Geometry: final body of the model. Coordinates: model frame, mm. A direction names the side the tool comes from. Coordinates: 2 decimals unless noted, no trailing zeros. Write each loop counter-clockwise with the first axis right and the second up, starting at its lowest first coordinate (ties: lowest second). Pieces come first, ordered by that corner, then holes. Notation, with made-up numbers: M 15,6 L 38,6 A28 cw 38,26 Z; hole C 85.25,-36 d2. An arc over 180 degrees is marked long. Write item = value, one per line. Start each with the question number.
Item 1: Pull-direction query (Z, two-part tool) for faces 6 (the flat face through (-119, 24, -155.575)), 7 (the flat face through (0, 19, 5)), 8 (the flat face through (-241.3, 5, -163)), 9 (the flat face through (-119, 22, -152.4)); classes: +Z half, -Z half, draft (parallel to the pull), parting line (faces both ways), or undercut.
Item 2: First-contact query: pin 1 Ø17.5 at (x, y) = (-103.5, 19) entering from -Z (3 decimals); pin 2 Ø3.5 at (y, z) = (39, -153.5) entering from +X (3 decimals); pin 3 Ø8.5 at (x, y) = (-228.6, 28.575) entering from +Z; pin 4 Ø1.5 at (x, y) = (-41, 23) entering from +Z (3 decimals). Flat tips, straight axial feed; report the tip coordinate or a pass-through.
Item 3: Reachability of faces 1 (the flat face through (-119, 3.175, -172)), 2 (the flat face through (-119, 24, 155.575)), 3 (the flat face through (20, 3.175, 5)), 4 (the flat face through (-119, 6.35, -173)), 5 (the flat face through (-119, 22, 152.4)) from +Z, -Z, +X, -X, +Y, -Y: full face, straight path, thin tool, end or side. Return the list, or none.
Item 4: Section B-B on z = 2.5. Output: boundary loops of the cut face in (x, y) (3 decimals), plus the area to 3 significant figures.
Item 5: Section A-A on x = -106.5. Output: boundary loops of the cut face in (y, z) (3 decimals).
Item 6: Ray query, L1, parallel to Z at x = -228.6, y = 4.1 (3 decimals); L2, parallel to Z at x = 25, y = 1; L3, parallel to Z at x = -209.5, y = 22 (3 decimals). Return the intervals inside material, ascending. Write a range as [from, to].
from build123d import *

# Parameters (mm, degrees)
EXTRUDE_THIN1_DEPTH     = 342.9
EXTRUDE_THIN2_DEPTH     = 241.3
CUT_EXTRUDE1_REACH      = 423.02
SKETCH3_R               = 3.175
CUT_EXTRUDE2_REACH      = 423.319
SKETCH4_R               = 3.175
CUT_EXTRUDE3_DEPTH      = 422.319030694
CUT_EXTRUDE3_DEPTH_BACK = 422.319030694
SKETCH5_R               = 4.7625


# Read off the part's stored shape, not the designer's step: Extrude-Thin2
with BuildPart() as part:
    # Sketch1 → Extrude-Thin1 (new, symmetric)
    with BuildSketch(Plane.XY):
        Polygon((38.1, 0), (0, 0), (0, 38.1), (3.175, 38.1), (3.175, 3.175), (38.1, 3.175), align=None)
    extrude(amount=EXTRUDE_THIN1_DEPTH, both=True)

    # Extrude-Thin2 outline → Extrude-Thin2 (add)
    with BuildSketch(Plane.ZY):
        Polygon((-152.4, 3.175), (-152.4, 41.275), (-155.575, 41.275), (-155.575, 6.35), (-190.5, 6.35), (-190.5, 3.175), align=None)
        Polygon((155.575, 6.35), (155.575, 41.275), (152.4, 41.275), (152.4, 3.175), (190.5, 3.175), (190.5, 6.35), align=None)
    extrude(amount=EXTRUDE_THIN2_DEPTH)

    # Sketch3 → Cut-Extrude1 (cut, up to next)
    with BuildSketch(Plane.XZ.offset(-3.175), mode=Mode.PRIVATE) as cut_extrude1_sk1:
        with Locations(Location((-228.6, 171.45, 0), (0, 0, 270))):
            Circle(SKETCH3_R)
    cut_extrude1_tool1 = extrude(cut_extrude1_sk1.sketch, amount=-CUT_EXTRUDE1_REACH, mode=Mode.PRIVATE) & part.part
    # Sketch3 → Cut-Extrude1 (cut, up to next)
    with BuildSketch(Plane.XZ.offset(-3.175), mode=Mode.PRIVATE) as cut_extrude1_sk2:
        with Locations(Location((-203.2, 171.45, 0), (0, 0, 270))):
            Circle(SKETCH3_R)
    cut_extrude1_tool2 = extrude(cut_extrude1_sk2.sketch, amount=-CUT_EXTRUDE1_REACH, mode=Mode.PRIVATE) & part.part
    # Sketch3 → Cut-Extrude1 (cut, up to next)
    with BuildSketch(Plane.XZ.offset(-3.175), mode=Mode.PRIVATE) as cut_extrude1_sk3:
        with Locations(Location((-228.6, -171.45, 0), (0, 0, 270))):
            Circle(SKETCH3_R)
    cut_extrude1_tool3 = extrude(cut_extrude1_sk3.sketch, amount=-CUT_EXTRUDE1_REACH, mode=Mode.PRIVATE) & part.part
    # Sketch3 → Cut-Extrude1 (cut, up to next)
    with BuildSketch(Plane.XZ.offset(-3.175), mode=Mode.PRIVATE) as cut_extrude1_sk4:
        with Locations(Location((-203.2, -171.45, 0), (0, 0, 270))):
            Circle(SKETCH3_R)
    cut_extrude1_tool4 = extrude(cut_extrude1_sk4.sketch, amount=-CUT_EXTRUDE1_REACH, mode=Mode.PRIVATE) & part.part
    add(cut_extrude1_tool1.solids().sort_by_distance((-228.6, 3.175, 171.45))[0], mode=Mode.SUBTRACT)
    add(cut_extrude1_tool2.solids().sort_by_distance((-203.2, 3.175, 171.45))[0], mode=Mode.SUBTRACT)
    add(cut_extrude1_tool3.solids().sort_by_distance((-228.6, 3.175, -171.45))[0], mode=Mode.SUBTRACT)
    add(cut_extrude1_tool4.solids().sort_by_distance((-203.2, 3.175, -171.45))[0], mode=Mode.SUBTRACT)

    # Sketch4 → Cut-Extrude2 (cut, up to next)
    with BuildSketch(Plane.XZ, mode=Mode.PRIVATE) as cut_extrude2_sk1:
        with Locations(Location((25.4, -336.55, 0), (0, 0, 270))):
            Circle(SKETCH4_R)
    cut_extrude2_tool1 = extrude(cut_extrude2_sk1.sketch, amount=-CUT_EXTRUDE2_REACH, mode=Mode.PRIVATE) & part.part
    # Sketch4 → Cut-Extrude2 (cut, up to next)
    with BuildSketch(Plane.XZ, mode=Mode.PRIVATE) as cut_extrude2_sk2:
        with Locations(Location((25.4, -273.05, 0), (0, 0, 270))):
            Circle(SKETCH4_R)
    cut_extrude2_tool2 = extrude(cut_extrude2_sk2.sketch, amount=-CUT_EXTRUDE2_REACH, mode=Mode.PRIVATE) & part.part
    # Sketch4 → Cut-Extrude2 (cut, up to next)
    with BuildSketch(Plane.XZ, mode=Mode.PRIVATE) as cut_extrude2_sk3:
        with Locations(Location((25.4, 273.05, 0), (0, 0, 270))):
            Circle(SKETCH4_R)
    cut_extrude2_tool3 = extrude(cut_extrude2_sk3.sketch, amount=-CUT_EXTRUDE2_REACH, mode=Mode.PRIVATE) & part.part
    # Sketch4 → Cut-Extrude2 (cut, up to next)
    with BuildSketch(Plane.XZ, mode=Mode.PRIVATE) as cut_extrude2_sk4:
        with Locations(Location((25.4, 336.55, 0), (0, 0, 270))):
            Circle(SKETCH4_R)
    cut_extrude2_tool4 = extrude(cut_extrude2_sk4.sketch, amount=-CUT_EXTRUDE2_REACH, mode=Mode.PRIVATE) & part.part
    add(cut_extrude2_tool1.solids().sort_by_distance((25.4, 0, -336.55))[0], mode=Mode.SUBTRACT)
    add(cut_extrude2_tool2.solids().sort_by_distance((25.4, 0, -273.05))[0], mode=Mode.SUBTRACT)
    add(cut_extrude2_tool3.solids().sort_by_distance((25.4, 0, 273.05))[0], mode=Mode.SUBTRACT)
    add(cut_extrude2_tool4.solids().sort_by_distance((25.4, 0, 336.55))[0], mode=Mode.SUBTRACT)

    # Sketch5 → Cut-Extrude3 (cut, two sides: drawn at the far end of the back side and taken through both)
    with BuildSketch(Plane.XY.offset(-CUT_EXTRUDE3_DEPTH_BACK)):
        with Locations((-228.6, 28.575)):
            Circle(SKETCH5_R)
        with Locations((-38.1, 28.575)):
            Circle(SKETCH5_R)
    extrude(amount=CUT_EXTRUDE3_DEPTH + CUT_EXTRUDE3_DEPTH_BACK, mode=Mode.SUBTRACT)


solid = part.part
Responses:
q1.face_6 = -Z half
q1.face_7 = undercut
q1.face_8 = draft
q1.face_9 = undercut
q2.pin_1 = -155.575
q2.pin_2 = 3.175
q2.pin_3 = through
q2.pin_4 = 155.575
q3.face_1 = +Z, -Z, -X, -Y
q3.face_2 = +Z, -X, +Y
q3.face_3 = +Z, -Z, +X, +Y
q3.face_4 = -Z, -X, +Y
q3.face_5 = -X, +Y, -Y
q4.outline = M 0,0 L 38.1,0 L 38.1,3.175 L 3.175,3.175 L 3.175,38.1 L 0,38.1 Z
q4.area = 232 mm²
q5.outline = M 3.175,-190.5 L 6.35,-190.5 L 6.35,-155.575 L 41.275,-155.575 L 41.275,-152.4 L 3.175,-152.4 Z; M 3.175,152.4 L 41.275,152.4 L 41.275,155.575 L 6.35,155.575 L 6.35,190.5 L 3.175,190.5 Z
q6.L1 = [-190.5, -174.625], [-168.275, -152.4], [152.4, 168.275], [174.625, 190.5]
q6.L2 = [-342.9, -339.7], [-333.4, -276.2], [-269.9, 269.9], [276.2, 333.4], [339.7, 342.9]
q6.L3 = [-155.575, -152.4], [152.4, 155.575]
